Geometry: final body of the model. Coordinates: model frame, mm. A direction names the side the tool comes from. Give positions to 0.01 mm unless a question says otherwise; leave off trailing zeros. Order: outer loops, then holes, each group sorted by start corner. A loop starts at its lowest first (then second) coordinate and runs counter-clockwise, first axis right, second up. Notation, with made-up numbers: (-26, 44) - (1, 44) arc R19 ccw to (1, 65) - close; hole circle Ø10 at (-11, 59). An arc over 180 degrees is marked (long way). Use one line per item in the form item = value.
from build123d import *

# Parameters (mm, degrees)
F1_W     = 52
F1_H     = 1.3
F1_H_2   = 5.6
F2_DEPTH = 1.5
F3_DEPTH = 7.4
F4_W     = 1.4
F4_H     = 1.5
F4_W_2   = 0.15
F4_W_3   = 1.25
F5_DEPTH = 5.9


with BuildPart() as f2:
    # F1 (on Top) → F2 (new body)
    with BuildSketch(Plane.XY):
        with Locations((26, -0.65)):
            Rectangle(F1_W, F1_H)
        with Locations((26, -4.1)):
            Rectangle(F1_W, F1_H_2)
        with Locations((26, -7.55)):
            Rectangle(F1_W, F1_H)
    extrude(amount=F2_DEPTH)

    # F1 (on Top) → F3 (join)
    with BuildSketch(Plane.XY):
        with Locations((26, -7.55)):
            Rectangle(F1_W, F1_H)
        with Locations((26, -0.65)):
            Rectangle(F1_W, F1_H)
    extrude(amount=F3_DEPTH)

    # F4 (on face) → F5 (join)
    with BuildSketch(Plane.XY.offset(1.5)):
        with Locations((0.7, -2.05)):
            Rectangle(F4_W, F4_H)
        with Locations((0.7, -6.15)):
            Rectangle(F4_W, F4_H)
        with Locations((3.675, -2.05)):
            Rectangle(F4_W_2, F4_H)
        with Locations((4.375, -2.05)):
            Rectangle(F4_W_3, F4_H)
        with Locations((5.075, -2.05)):
            Rectangle(F4_W_2, F4_H)
        with Locations((3.675, -6.15)):
            Rectangle(F4_W_2, F4_H)
        with Locations((4.375, -6.15)):
            Rectangle(F4_W_3, F4_H)
        with Locations((5.075, -6.15)):
            Rectangle(F4_W_2, F4_H)
        with Locations((7.425, -2.05)):
            Rectangle(F4_W_2, F4_H)
        with Locations((8.125, -2.05)):
            Rectangle(F4_W_3, F4_H)
        with Locations((8.825, -2.05)):
            Rectangle(F4_W_2, F4_H)
        with Locations((7.425, -6.15)):
            Rectangle(F4_W_2, F4_H)
        with Locations((8.125, -6.15)):
            Rectangle(F4_W_3, F4_H)
        with Locations((8.825, -6.15)):
            Rectangle(F4_W_2, F4_H)
        with Locations((11.175, -2.05)):
            Rectangle(F4_W_2, F4_H)
        with Locations((11.875, -2.05)):
            Rectangle(F4_W_3, F4_H)
        with Locations((12.575, -2.05)):
            Rectangle(F4_W_2, F4_H)
        with Locations((11.175, -6.15)):
            Rectangle(F4_W_2, F4_H)
        with Locations((11.875, -6.15)):
            Rectangle(F4_W_3, F4_H)
        with Locations((12.575, -6.15)):
            Rectangle(F4_W_2, F4_H)
        with Locations((14.925, -2.05)):
            Rectangle(F4_W_2, F4_H)
        with Locations((15.625, -2.05)):
            Rectangle(F4_W_3, F4_H)
        with Locations((16.325, -2.05)):
            Rectangle(F4_W_2, F4_H)
        with Locations((14.925, -6.15)):
            Rectangle(F4_W_2, F4_H)
        with Locations((15.625, -6.15)):
            Rectangle(F4_W_3, F4_H)
        with Locations((16.325, -6.15)):
            Rectangle(F4_W_2, F4_H)
        with Locations((18.675, -2.05)):
            Rectangle(F4_W_2, F4_H)
        with Locations((19.375, -2.05)):
            Rectangle(F4_W_3, F4_H)
        with Locations((20.075, -2.05)):
            Rectangle(F4_W_2, F4_H)
        with Locations((18.675, -6.15)):
            Rectangle(F4_W_2, F4_H)
        with Locations((19.375, -6.15)):
            Rectangle(F4_W_3, F4_H)
        with Locations((20.075, -6.15)):
            Rectangle(F4_W_2, F4_H)
        with Locations((22.425, -2.05)):
            Rectangle(F4_W_2, F4_H)
        with Locations((23.125, -2.05)):
            Rectangle(F4_W_3, F4_H)
        with Locations((23.825, -2.05)):
            Rectangle(F4_W_2, F4_H)
        with Locations((22.425, -6.15)):
            Rectangle(F4_W_2, F4_H)
        with Locations((23.125, -6.15)):
            Rectangle(F4_W_3, F4_H)
        with Locations((23.825, -6.15)):
            Rectangle(F4_W_2, F4_H)
        with Locations((26.175, -2.05)):
            Rectangle(F4_W_2, F4_H)
        with Locations((26.875, -2.05)):
            Rectangle(F4_W_3, F4_H)
        with Locations((27.575, -2.05)):
            Rectangle(F4_W_2, F4_H)
        with Locations((26.175, -6.15)):
            Rectangle(F4_W_2, F4_H)
        with Locations((26.875, -6.15)):
            Rectangle(F4_W_3, F4_H)
        with Locations((27.575, -6.15)):
            Rectangle(F4_W_2, F4_H)
        with Locations((29.925, -2.05)):
            Rectangle(F4_W_2, F4_H)
        with Locations((30.625, -2.05)):
            Rectangle(F4_W_3, F4_H)
        with Locations((31.325, -2.05)):
            Rectangle(F4_W_2, F4_H)
        with Locations((29.925, -6.15)):
            Rectangle(F4_W_2, F4_H)
        with Locations((30.625, -6.15)):
            Rectangle(F4_W_3, F4_H)
        with Locations((31.325, -6.15)):
            Rectangle(F4_W_2, F4_H)
        with Locations((33.675, -2.05)):
            Rectangle(F4_W_2, F4_H)
        with Locations((34.375, -2.05)):
            Rectangle(F4_W_3, F4_H)
        with Locations((35.075, -2.05)):
            Rectangle(F4_W_2, F4_H)
        with Locations((33.675, -6.15)):
            Rectangle(F4_W_2, F4_H)
        with Locations((34.375, -6.15)):
            Rectangle(F4_W_3, F4_H)
        with Locations((35.075, -6.15)):
            Rectangle(F4_W_2, F4_H)
        with Locations((37.425, -2.05)):
            Rectangle(F4_W_2, F4_H)
        with Locations((38.125, -2.05)):
            Rectangle(F4_W_3, F4_H)
        with Locations((38.825, -2.05)):
            Rectangle(F4_W_2, F4_H)
        with Locations((37.425, -6.15)):
            Rectangle(F4_W_2, F4_H)
        with Locations((38.125, -6.15)):
            Rectangle(F4_W_3, F4_H)
        with Locations((38.825, -6.15)):
            Rectangle(F4_W_2, F4_H)
        with Locations((41.175, -2.05)):
            Rectangle(F4_W_2, F4_H)
        with Locations((41.875, -2.05)):
            Rectangle(F4_W_3, F4_H)
        with Locations((42.575, -2.05)):
            Rectangle(F4_W_2, F4_H)
        with Locations((41.175, -6.15)):
            Rectangle(F4_W_2, F4_H)
        with Locations((41.875, -6.15)):
            Rectangle(F4_W_3, F4_H)
        with Locations((42.575, -6.15)):
            Rectangle(F4_W_2, F4_H)
        with Locations((44.925, -2.05)):
            Rectangle(F4_W_2, F4_H)
        with Locations((45.625, -2.05)):
            Rectangle(F4_W_3, F4_H)
        with Locations((46.325, -2.05)):
            Rectangle(F4_W_2, F4_H)
        with Locations((44.925, -6.15)):
            Rectangle(F4_W_2, F4_H)
        with Locations((45.625, -6.15)):
            Rectangle(F4_W_3, F4_H)
        with Locations((46.325, -6.15)):
            Rectangle(F4_W_2, F4_H)
        with Locations((49.3, -2.05)):
            Rectangle(F4_W, F4_H)
        with Locations((49.3, -6.15)):
            Rectangle(F4_W, F4_H)
    extrude(amount=F5_DEPTH)


solid = f2.part
(1) Cut plane A-A on x = 32.5. Output: boundary loops of the cut face in (y, z).
Computed values:
outline = (-8.2, 0) - (0, 0) - (0, 7.4) - (-1.3, 7.4) - (-1.3, 1.5) - (-6.9, 1.5) - (-6.9, 7.4) - (-8.2, 7.4) - close
(2) Pull-direction query (X, two-part tool) for faces 1 (the face through (23, -2.8, 4)), 2 (the face through (42.65, -6, 4)); classes: released by +X, released by -X, zero draft, split by the parting line, or undercut.
Computed values:
face_1 = zero draft
face_2 = undercut
(3) Reachability of faces 3 (the face through (25.6, -7.1, 7.4)), 4 (the face through (27, -2.8, 4)), 5 (the face through (11.1, -6, 4)) from +Z, -Z, +X, -X, +Y, -Y: full face, straight path, thin tool, end or side. Return the list, or none.
Computed values:
face_3 = +Z, +X, -X, +Y, -Y
face_4 = +Z, +X, -X
face_5 = +Z
(4) Cut plane B-B on y = -4.25. Output: boundary loops of the cut face in (x, z).
Computed values:
outline = (0, 0) - (52, 0) - (52, 1.5) - (0, 1.5) - close
(5) Ray query, line 1 along Y through (x, z) = (21, 4); line 2 along Y through (x, z) = (4, 5.75); line 3 along Z through (x, y) = (43, -3.25). Return the intervals inside material, ascending.
Computed values:
line_1 = -8.2 to -6.9, -1.3 to 0
line_2 = -8.2 to -5.4, -2.8 to 0
line_3 = 0 to 1.5
